Verification items for the finished model (mm, model axes). Give positions to 0.01 mm unless a question says otherwise; leave off trailing zeros. Write each loop counter-clockwise with the first axis right and the second up, starting at its lowest first coordinate (ties: lowest second). Pieces come first, ordered by that corner, then holes. Notation, with made-up numbers: (14.25, 85) - (46.25, 85) arc R9 cw to (46.25, 95) - close; hole circle Ø6 at (41.25, -20). An arc over 180 degrees is marked (long way). Answer as a JSON object with one key per item and string values. Group by question number.
Item 1: Scan lines: line 1 along X through (y, z) = (-11, 10.25); line 2 along X through (y, z) = (-18.5, 9.25). Record each from-to range of solid material in increasing order. Write a range as [from, to].
Item 2: Sectioned sample at B-B, the plane y = -16.5. Record the boundary of the cut face in (x, z) (3 decimals).
Item 3: Sectioned sample at A-A, the plane x = 24. Record the boundary of the cut face in (y, z) (3 decimals).
Item 4: Sectioned sample at C-C, the plane z = 14.5. Record the boundary of the cut face in (x, y), and give its area (3 significant figures).
Item 5: Draft check along X on faces 1 (the face through (-58.641, 0, 11)), 2 (the face through (28.105, -18.751, 11.268)), 3 (the face through (16, 1, 0)). Enter one of: +X half, -X half, draft (parallel to the pull), parting line (faces both ways), or undercut.
Autodesk Inventor part; units mm, degrees
ref_plane "YZ Plane" through (0, 0, 0) normal (1, 0, 0) x (0, 1, 0)
ref_plane "XZ Plane" through (0, 0, 0) normal (0, 1, 0) x (-1, 0, 0)
ref_plane "XY Plane" through (0, 0, 0) normal (0, 0, 1) x (1, 0, 0)
sketch "Sketch1" plane through (0, 0, 0) normal (0, 0, 1) x (1, 0, 0)
  line L0 (-58.6409, 36.9404) -> (93.7591, 36.9404)
  line L1 (93.7591, 36.9404) -> (93.7591, -36.0846)
  line L2 (93.7591, -36.0846) -> (-58.6409, -36.0846)
  line L3 (-58.6409, -36.0846) -> (-58.6409, 36.9404)
  point P0 (0, 0)
  dimension "d0" = 152.4
  dimension "d1" = 73.025
extrude "Extrusion1" add sketch "Sketch1" along normal blind 22.225
sketch "Sketch2" plane through (0, 0, 22.225) normal (0, 0, 1) x (1, 0, 0)
  line L0 (-58.6409, 36.9404) -> (-58.6409, -36.0846)
  line L1 (-58.6409, -36.0846) -> (93.7591, -36.0846)
  circle A0 centre (23.9091, -10.6846) radius 9.092
  point P0 (0, 0)
  dimension "d4" = 82.55
  dimension "d5" = 25.4
extrude "Extrusion2" cut sketch "Sketch2" against normal blind 22.225
properties part number "FrameEndSpacer_NERDS"
Geometry check:
{
 "1": {"line 1": "[-58.64, 14.82], [33, 93.76]", "line 2": "[-58.64, 19.26], [28.55, 93.76]"},
 "2": {"outline": "(-58.641, 0) - (16.92, 0) - (16.92, 22.225) - (-58.641, 22.225) - close; (30.898, 0) - (93.759, 0) - (93.759, 22.225) - (30.898, 22.225) - close"},
 "3": {"outline": "(-36.085, 0) - (-19.776, 0) - (-19.776, 22.225) - (-36.085, 22.225) - close; (-1.593, 0) - (36.94, 0) - (36.94, 22.225) - (-1.593, 22.225) - close"},
 "4": {"outline": "(-58.64, -36.08) - (93.76, -36.08) - (93.76, 36.94) - (-58.64, 36.94) - close; hole circle Ø18.18 at (23.91, -10.68)", "area": "10,900 mm^2"},
 "5": {"face 1": "-X half", "face 2": "undercut", "face 3": "draft"}
}
